from build123d import *

# Parameters (mm, degrees)
F1_DEPTH = 6
F2_DEPTH = 11
F3_DEPTH = 8
F4_DEPTH = 3


# Not quite as in the source:
# - a feature names something its author has since deleted; it is built from what else it names


with BuildPart() as f1:
    # F0 (on Top) → F1 (new body)
    with BuildSketch(Plane.XY):
        with BuildLine():
            Line((48.7961772168, 43.654083433), (48.941615093, 44.8955937326))
            ThreePointArc((48.941615093, 44.8955937326), (46.1510840758, 42.4540888757), (48.8589984809, 39.9212626086))
            Line((48.8589984809, 39.9212626086), (48.7548689108, 41.1669178709))
            ThreePointArc((48.7548689108, 41.1669178709), (47.4009117082, 42.4333310045), (48.7961772168, 43.654083433))
        make_face()
        with BuildLine():
            ThreePointArc((51.1507393406, 42.4125731333), (50.5185173495, 44.0743208005), (48.941615093, 44.8955937326))
            Line((48.941615093, 44.8955937326), (48.7961772168, 43.654083433))
            ThreePointArc((48.7961772168, 43.654083433), (49.5846283451, 43.2434469669), (49.9007393406, 42.4125731333))
            ThreePointArc((49.9007393406, 42.4125731333), (49.5707018297, 41.5663054341), (48.7548689108, 41.1669178709))
            Line((48.7548689108, 41.1669178709), (48.8589984809, 39.9212626086))
            ThreePointArc((48.8589984809, 39.9212626086), (50.4906643188, 40.7200377349), (51.1507393406, 42.4125731333))
        make_face()
    extrude(amount=F1_DEPTH)

    # F0 (on Top) → F2 (join)
    with BuildSketch(Plane.XY):
        with BuildLine():
            ThreePointArc((49.9007393406, 42.4125731333), (49.5846283451, 43.2434469669), (48.7961772168, 43.654083433))
            Line((48.7961772168, 43.654083433), (48.6507393406, 42.4125731333))
            Line((48.6507393406, 42.4125731333), (48.7548689108, 41.1669178709))
            ThreePointArc((48.7548689108, 41.1669178709), (49.5707018297, 41.5663054341), (49.9007393406, 42.4125731333))
        make_face()
        with BuildLine():
            Line((48.6507393406, 42.4125731333), (48.7961772168, 43.654083433))
            ThreePointArc((48.7961772168, 43.654083433), (47.4009117082, 42.4333310045), (48.7548689108, 41.1669178709))
            Line((48.7548689108, 41.1669178709), (48.6507393406, 42.4125731333))
        make_face()
    extrude(amount=F2_DEPTH)



with BuildPart() as f3:
    # F0 (on Top) → F3 (new body)
    with BuildSketch(Plane.XY):
        with BuildLine():
            Line((53.5294346637, 82.6926567151), (53.515810825, 83.9425824693))
            Line((53.515810825, 83.9425824693), (53.3703729488, 82.7010721697))
            ThreePointArc((53.3703729488, 82.7010721697), (53.4497696251, 82.6943282645), (53.5294346637, 82.6926567151))
        make_face()
        with BuildLine():
            Line((53.3703729488, 82.7010721697), (53.515810825, 83.9425824693))
            Line((53.515810825, 83.9425824693), (53.5294346637, 82.6926567151))
            ThreePointArc((53.5294346637, 82.6926567151), (54.4044980024, 83.0635289438), (54.765810825, 83.9425824693))
            ThreePointArc((54.765810825, 83.9425824693), (54.7657365792, 83.9562063081), (54.7655138506, 83.9698285284))
            ThreePointArc((54.7655138506, 83.9698285284), (53.5021869863, 85.1925082235), (52.265810825, 83.9425824693))
            ThreePointArc((52.265810825, 83.9425824693), (52.5819218206, 83.1117086357), (53.3703729488, 82.7010721697))
        make_face()
    extrude(amount=F3_DEPTH)


with BuildPart() as f1_1:
    add(f1.part)

    add(f3.part)  # F4 merges F3
    # F0 (on Top) → F4 (join)
    with BuildSketch(Plane.XY):
        with BuildLine():
            ThreePointArc((54.765810825, 83.9425824693), (54.4044980024, 83.0635289438), (53.5294346637, 82.6926567151))
            Line((53.5294346637, 82.6926567151), (54.7385631476, -28.239428033))
            ThreePointArc((54.7385631476, -28.239428033), (56.5044417212, -28.9428490232), (57.2652168763, -30.6847874233))
            Line((57.2652168763, -30.6847874233), (54.7655138506, 83.9698285284))
            ThreePointArc((54.7655138506, 83.9698285284), (54.7657365792, 83.9562063081), (54.765810825, 83.9425824693))
        make_face()
        with BuildLine():
            Line((54.7385631476, -28.239428033), (53.5294346637, 82.6926567151))
            ThreePointArc((53.5294346637, 82.6926567151), (53.4497696251, 82.6943282645), (53.3703729488, 82.7010721697))
            Line((53.3703729488, 82.7010721697), (52.265810825, 73.2721304859))
            Line((52.265810825, 73.2721304859), (52.265810825, -0.8329027879))
            Line((52.265810825, -0.8329027879), (54.5575516847, -28.2479690167))
            ThreePointArc((54.5575516847, -28.2479690167), (54.6479800039, -28.2420579057), (54.7385631476, -28.239428033))
        make_face()
        with BuildLine():
            Line((52.265810825, 73.2721304859), (53.3703729488, 82.7010721697))
            ThreePointArc((53.3703729488, 82.7010721697), (52.5819218206, 83.1117086357), (52.265810825, 83.9425824693))
            Line((52.265810825, 83.9425824693), (52.265810825, 73.2721304859))
        make_face()
        with BuildLine():
            ThreePointArc((57.2652168763, -30.6847874233), (56.5044417212, -28.9428490232), (54.7385631476, -28.239428033))
            Line((54.7385631476, -28.239428033), (54.765810825, -30.7392795414))
            Line((54.765810825, -30.7392795414), (54.5575516847, -28.2479690167))
            ThreePointArc((54.5575516847, -28.2479690167), (52.9258858468, -29.0467441431), (52.265810825, -30.7392795414))
            ThreePointArc((52.265810825, -30.7392795414), (54.765810825, -33.2392795414), (57.265810825, -30.7392795414))
            ThreePointArc((57.265810825, -30.7392795414), (57.2656623334, -30.712031864), (57.2652168763, -30.6847874233))
        make_face()
        with BuildLine():
            Line((54.765810825, -30.7392795414), (54.7385631476, -28.239428033))
            ThreePointArc((54.7385631476, -28.239428033), (54.6479800039, -28.2420579057), (54.5575516847, -28.2479690167))
            Line((54.5575516847, -28.2479690167), (54.765810825, -30.7392795414))
        make_face()
        with BuildLine():
            Line((52.265810825, -0.8329027879), (52.265810825, 73.2721304859))
            Line((52.265810825, 73.2721304859), (48.941615093, 44.8955937326))
            ThreePointArc((48.941615093, 44.8955937326), (50.5185173495, 44.0743208005), (51.1507393406, 42.4125731333))
            ThreePointArc((51.1507393406, 42.4125731333), (50.4906643188, 40.7200377349), (48.8589984809, 39.9212626086))
            Line((48.8589984809, 39.9212626086), (52.265810825, -0.8329027879))
        make_face()
        with BuildLine():
            ThreePointArc((52.265810825, -30.7392795414), (52.9258858468, -29.0467441431), (54.5575516847, -28.2479690167))
            Line((54.5575516847, -28.2479690167), (52.265810825, -0.8329027879))
            Line((52.265810825, -0.8329027879), (52.265810825, -30.7392795414))
        make_face()
    extrude(amount=F4_DEPTH)


solid = f1_1.part
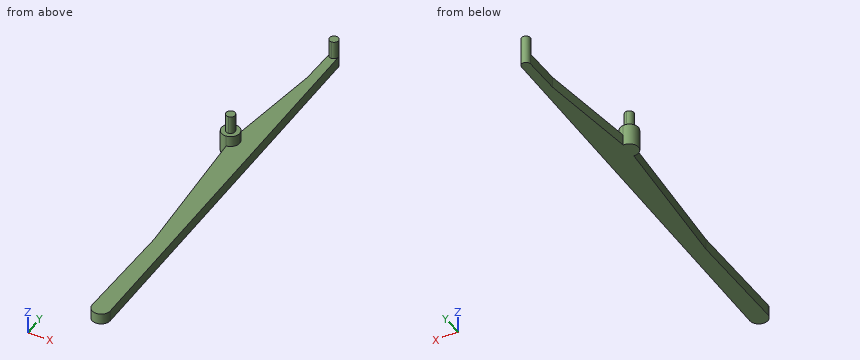
Could you check a few things on this model? Use its own coordinates, in mm. Give positions to 0.01 mm unless a question says otherwise; leave off trailing zeros. Write each loop counter-clockwise with the first axis right and the second up, starting at its lowest first coordinate (ties: lowest second). Pieces come first, ordered by that corner, then holes. Notation, with made-up numbers: (63.5, 27.25) -> (105.5, 27.25) arc R29 cw to (105.5, 59.25) -> close; hole circle Ø4 at (-3.5, -24.75). An arc over 180 degrees is marked (long way). Answer as CSV lines item,"result". Start each with the question number.
(1) If we section it at A-A, the plane z = 1.75: Write out the boundary of the cut face in (x, y), and give its area (3 significant figures).
(2) I'm going to push flat-ended pins straight in: pin 1 Ø3.5 at (y, z) = (80, 2) entering from -X; pin 2 Ø2 at (y, z) = (5.5, 3) entering from +X; pin 3 Ø4 at (x, z) = (53.5, 9) entering from -Y; pin 4 Ø6 at (x, z) = (55, 4.5) entering from +Y. Where does each tip first touch, or does it pass through?
(3) If we section it at D-D, the plane z = 9: Write out the boundary of the cut face in (x, y), and give its area (3 significant figures).
(4) If we section it at C-C, the plane x = 56: Write out the boundary of the cut face in (y, z), and give its area (3 significant figures).
(5) Please list where these lines run through material, in increasing order: line 1 (Z direction, x = 53, y = -16.5); line 2 (Y direction, x = 48.5, z = 3.75); line 3 (X direction, y = -25, z = 0.5).
(6) If we section it at B-B, the plane y = -8: Write out the boundary of the cut face in (x, z).
Answer list:
1,outline,"(48.86, 39.92) -> (52.27, -0.83) -> (52.27, -30.74) arc R2.5 ccw (long way) to (57.27, -30.68) -> (54.77, 83.97) arc R1.25 ccw to (52.27, 83.94) -> (52.27, 73.27) -> (48.94, 44.9) arc R2.5 ccw (long way) to start"
1,area,"587 mm^2"
2,pin 1,"x = 52.27"
2,pin 2,"x = 56.5"
2,pin 3,"y = 82.69"
2,pin 4,"y = 85.19"
3,outline,"circle Ø2.5 at (48.65, 42.41)"
3,area,"4.91 mm^2"
4,outline,"(-32.91, 0) -> (27.35, 0) -> (27.35, 3) -> (-32.91, 3) -> close"
4,area,"181 mm^2"
5,line 1,"0 to 3"
5,line 2,"39.92 to 44.91"
5,line 3,"52.27 to 57.14"
6,outline,"(52.27, 0) -> (56.77, 0) -> (56.77, 3) -> (52.27, 3) -> close"
